Can you work these out from the model? Positions are in its coordinate system, mm. Face numbers are marked on the shaded views. A direction names the side the tool comes from. Round coordinates to 2 decimals unless told otherwise and drop trailing zeros. Order: outer loops, then holes, each group sorted by start corner. A loop starts at its lowest first (then second) coordinate and runs counter-clockwise, first axis right, second up.
Q1. We'd pull the mould along X, two halves only. Please class the marked faces 4, 5 and 6: pulls with the +X half, pulls with the -X half, needs draft (parallel to the pull), parting line crosses it, or undercut.
Q2. Will these pins go through, and if not, where does the flat tip stop? P1, Ø0.8, axis at x = 11, y = 1, coming from the +Z side; P2, Ø1.5, axis at y = 1, z = 12.5, coming from the -X side; P3, Ø1, axis at x = -8, y = 2, coming from the -Z side.
Q3. If we section it at A-A (z = 13.75): Please give me the cut outline in (x, y).
Q4. If I drill on line 1 (Z direction, x = 0, y = 0.95); line 2 (X direction, y = 1.8, z = 0); line 3 (X direction, y = 0.35, z = 12.5), over which ranges is the centre line in solid material (lowest first)?
Q5. For the marked faces 1, 2 and 3, which set-ups out of +Z, -Z, +X, -X, +Y, -Y let a thin tool reach every point of the face, with its end or its side?
Q6. If we section it at D-D (x = -8.75): Please give me the cut outline in (y, z), plus the area to 3 significant figures.
Q7. If we section it at B-B (x = 0): Please give me the cut outline in (y, z), plus the area to 3 significant figures.
Q8. If we section it at C-C (y = 0.3): Please give me the cut outline in (x, z), plus the area to 3 significant figures.
from build123d import *

# Parameters (mm, degrees)
BOSS_EXTRUDE1_DEPTH = 3
SKETCH3_R           = 1.5
CUT_EXTRUDE1_DEPTH  = 3
FILLET1_R           = 2
FILLET2_R           = 0.5


with BuildPart() as part:
    # Sketch2 → Boss-Extrude1 (new body)
    with BuildSketch(Plane(origin=(0, 0, 0), x_dir=(1, 0, 0), z_dir=(0, 1, 0))):
        with BuildLine():
            Line((-11.531388224, -10.806413351), (-10.031388224, -10.806413351))
            Line((-10.031388224, -10.806413351), (-10.031388224, -14.806413351))
            Line((-10.031388224, -14.806413351), (-4.231388224, -14.806413351))
            Line((-4.231388224, -14.806413351), (-4.231388224, -10.806413351))
            Line((-4.231388224, -10.806413351), (-0.781388224, -10.806413351))
            Line((-0.781388224, -10.806413351), (-0.781388224, -6.306413351))
            Line((-0.781388224, -6.306413351), (1.218611776, -6.306413351))
            Line((1.218611776, -6.306413351), (1.218611776, -10.806413351))
            Line((1.218611776, -10.806413351), (4.668611776, -10.806413351))
            Line((4.668611776, -10.806413351), (4.668611776, -14.59443044))
            Line((4.668611776, -14.59443044), (10.468611776, -14.59443044))
            Line((10.468611776, -14.59443044), (10.468611776, -10.59443044))
            Line((10.468611776, -10.59443044), (11.968611776, -10.59443044))
            Line((11.968611776, -10.59443044), (11.968611776, -5.761851858))
            ThreePointArc((11.968611776, -5.761851858), (7.254363967, -4.368466387), (5, 0))
            ThreePointArc((5, 0), (0, 5), (-5, 0))
            ThreePointArc((-5, 0), (-7.028472422, -4.339612176), (-11.531388224, -5.973834769))
            Line((-11.531388224, -5.973834769), (-11.531388224, -10.806413351))
        make_face()
    extrude(amount=BOSS_EXTRUDE1_DEPTH)

    # Sketch3 → Cut-Extrude1 (cut)
    with BuildSketch(Plane(origin=(0, 3, 0), x_dir=(1, 0, 0), z_dir=(0, 1, 0))):
        Circle(SKETCH3_R)
    extrude(amount=-CUT_EXTRUDE1_DEPTH, mode=Mode.SUBTRACT)

    # Fillet1
    fillet1_edges = [part.edges().sort_by_distance(p)[0] for p in [
        (11.968611776, 1.5, 5.761851858),
        (-11.531388224, 1.5, 5.973834769),
    ]]
    fillet(fillet1_edges, radius=FILLET1_R)

    # Fillet2
    fillet2_edges = [part.edges().sort_by_distance(p)[0] for p in [
        (10.468611776, 1.5, 14.59443044),
        (1.218611776, 1.5, 6.306413351),
        (-0.781388224, 1.5, 6.306413351),
        (-10.031388224, 1.5, 14.806413351),
    ]]
    fillet(fillet2_edges, radius=FILLET2_R)


solid = part.part
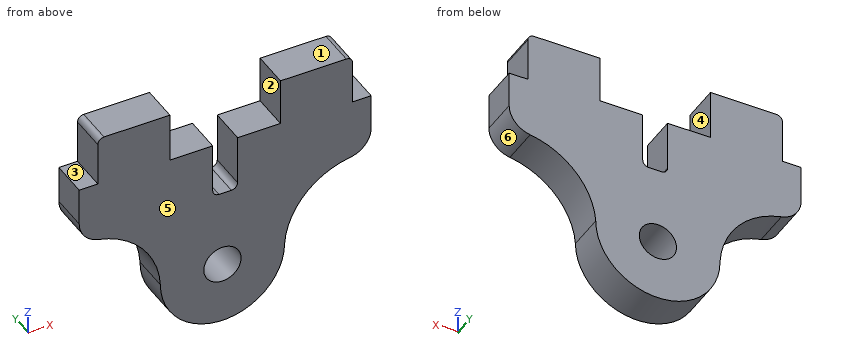
Solution:
1. face 4: undercut
1. face 5: needs draft
1. face 6: pulls with the +X half
2. P1: stops at z = 10.59
2. P2: stops at x = -10.03
2. P3: stops at z = 4.73
3. outline: (-10.03, 0) - (-4.23, 0) - (-4.23, 3) - (-10.03, 3) - close; (4.67, 0) - (10.47, 0) - (10.47, 3) - (4.67, 3) - close
4. line 1: z = -5 to -1.5, 1.5 to 6.31
4. line 2: x = -5 to -1.5, 1.5 to 5
4. line 3: x = -10.03 to -4.23, 4.67 to 10.47
5. face 1: +Z, +X, +Y, -Y
5. face 2: +Z, +Y, -Y
5. face 3: +Z, -X, +Y, -Y
6. outline: (0, 5.46) - (3, 5.46) - (3, 14.81) - (0, 14.81) - close
6. area: 28.0 mm2
7. outline: (0, -5) - (3, -5) - (3, -1.5) - (0, -1.5) - close; (0, 1.5) - (3, 1.5) - (3, 6.31) - (0, 6.31) - close
7. area: 24.9 mm2
8. outline: (-11.53, 7.8) arc R2 ccw to (-9.95, 5.84) arc R6.26 cw to (-5, 0) arc R5 ccw to (5, 0) arc R6.26 cw to (10.28, 5.73) arc R2 ccw to (11.97, 7.71) - (11.97, 10.59) - (10.47, 10.59) - (10.47, 14.09) arc R0.5 ccw to (9.97, 14.59) - (4.67, 14.59) - (4.67, 10.81) - (1.22, 10.81) - (1.22, 6.81) arc R0.5 cw to (0.72, 6.31) - (-0.28, 6.31) arc R0.5 cw to (-0.78, 6.81) - (-0.78, 10.81) - (-4.23, 10.81) - (-4.23, 14.81) - (-9.53, 14.81) arc R0.5 ccw to (-10.03, 14.31) - (-10.03, 10.81) - (-11.53, 10.81) - close; hole circle Ø3 at (0, 0)
8. area: 258 mm2
